Input: part model. Units: mm. Frame: model coordinates. A direction names the side the tool comes from. Coordinates: 2 decimals unless noted, no trailing zeros. Order: outer loops, then holes, each group sorted by start corner. A loop starts at its lowest first (then second) coordinate and runs counter-clockwise, first axis right, second up.
from build123d import *

# Parameters (mm, degrees)
BOSS_EXTRU_1_DEPTH      = 4
CONG_1_R                = 10
ESQUISSE3_R             = 1.55
ENL_V_MAT_EXTRU_1_DEPTH = 10


with BuildPart() as part:
    # Esquisse2 → Boss.-Extru.1 (new body)
    with BuildSketch(Plane(origin=(0, 0, 0), x_dir=(1, 0, 0), z_dir=(0, 1, 0))):
        Polygon((-15, 4.125844984), (-15, 7), (-5, 7), (-5, 0), (5, 0), (5, 7), (15, 7), (15, 0.999487428), (15, -20), (-15, -20), align=None)
    extrude(amount=BOSS_EXTRU_1_DEPTH)

    # Congé1
    cong_1_edges = [part.edges().sort_by_distance(p)[0] for p in [
        (15, 2, 20),
        (-15, 2, 20),
    ]]
    fillet(cong_1_edges, radius=CONG_1_R)

    # Esquisse3 → Enlèv. mat.-Extru.1 (cut)
    with BuildSketch(Plane(origin=(0, 4, 0), x_dir=(1, 0, 0), z_dir=(0, 1, 0))):
        with Locations(Location((5.483505043, -16.969125841, 0), (0, 0, 270))):
            Circle(ESQUISSE3_R)
        with Locations(Location((-4.516494957, -16.969125841, 0), (0, 0, 270))):
            Circle(ESQUISSE3_R)
    extrude(amount=-ENL_V_MAT_EXTRU_1_DEPTH, mode=Mode.SUBTRACT)


solid = part.part
Item 1: Access query for faces 1 (the face through (-12.15, 2.03, 16.99)), 2 (the face through (5, 2, -3)). Directions: +Z, -Z, +X, -X, +Y, -Y. A direction counts if a zero-diameter tool reaches every point of the face in a straight line with its end or side. Return the directions, or none.
Response values:
face 1: +Z, -X, +Y, -Y
face 2: -Z, +Y, -Y
Item 2: Pin query (flat end, axial travel): pin 1 Ø1.5 at (x, y) = (8, 2) entering from +Z; pin 2 Ø2 at (x, y) = (-1.5, 1.5) entering from -Z; pin 3 Ø1 at (y, z) = (1, 17) entering from -X. Return the tip coordinate at first contact, or that it passes through.
Response values:
pin 1: stops at z = 19.74
pin 2: stops at z = 0
pin 3: stops at x = -12.6
Item 3: Cut plane B-B on x = 6. Return loops of the section in (y, z), then the cut area to 3 significant figures.
Response values:
outline: (0, -7) - (4, -7) - (4, 15.51) - (0, 15.51) - close; (0, 18.43) - (4, 18.43) - (4, 19.95) - (0, 19.95) - close
area: 96.1 mm2
Item 4: Draft query along X for faces 3 (the face through (-5, 2, -4)), 4 (the face through (0, 4, 6)), 5 (the face through (15, 2, 2)). Return one class per face: pulls with the +X half, pulls with the -X half, needs draft (parallel to the pull), parting line crosses it, or undercut.
Response values:
face 3: undercut
face 4: needs draft
face 5: pulls with the +X half
Item 5: Cut plane A-A on z = -3.25. Return loops of the section in (x, y), then the cut area to 3 significant figures.
Response values:
outline: (-15, 0) - (-5, 0) - (-5, 4) - (-15, 4) - close; (5, 0) - (15, 0) - (15, 4) - (5, 4) - close
area: 80.0 mm2
Item 6: Cut plane D-D on x = -1. Return loops of the section in (y, z), then the cut area to 3 significant figures.
Response values:
outline: (0, 0) - (4, 0) - (4, 20) - (0, 20) - close
area: 80.0 mm2
Item 7: Ray query, probe 1 along X at (y, z) = (2.5, 15.75); probe 2 along X at (y, z) = (1.75, -5); probe 3 along Z at (x, y) = (-2, 3.3). Return the intervals inside material, ascending.
Response values:
probe 1: x = -13.18 to -5.47, -3.56 to 4.53, 6.44 to 13.18
probe 2: x = -15 to -5, 5 to 15
probe 3: z = 0 to 20
Item 8: Cut plane C-C on y = 2.4. Return loops of the section in (x, z), then the cut area to 3 significant figures.
Response values:
outline: (-15, -7) - (-5, -7) - (-5, 0) - (5, 0) - (5, -7) - (15, -7) - (15, 10) arc R10 ccw to (5, 20) - (-5, 20) arc R10 ccw to (-15, 10) - close; hole circle Ø3.1 at (-4.52, 16.97); hole circle Ø3.1 at (5.48, 16.97)
area: 682 mm2
